Source: CAD feature listing. Evaluate the final solid. Frame: model axes, mm. A direction names the side the tool comes from. Coordinates: 2 decimals unless noted, no trailing zeros. Write each loop counter-clockwise with the first axis right and the second up, starting at its lowest first coordinate (ties: lowest second). Pieces come first, ordered by that corner, then holes. Notation, with made-up numbers: M -13,79.5 L 42,79.5 A5 ccw 42,87.5 Z; hole C 61,64 d6. An arc over 180 degrees is marked long. One line per item, written item: value. Start each with the question number.
Item 1: Set-up query: faces 3 (the flat face through (2.5, 7, 0)), 4 (the cylindrical face through (-1.494, 4.107, -10.965)), 5 (the cylindrical face through (55.608, -59.05, -11.462)). Return all of +Z, -Z, +X, -X, +Y, -Y with unobstructed straight access to the full face (end or side cutting, diameter ignored); none if empty.
Item 2: Ray query, L1, parallel to Y at x = 74.5, z = 15.5; L2, parallel to X at y = 37.5, z = -2; L3, parallel to Y at x = 18, z = -20. Return the intervals inside material, ascending. Write a range as from..to.
Item 3: Cut plane C-C, the plane x = 49. Output: boundary loops of the cut face in (y, z), then the cut area to 3 significant figures.
Item 4: Pin query (flat end, axial travel): P1, Ø3, axis at y = 7.5, z = 11.5, coming from the -X side; P2, Ø5, axis at x = 21.5, z = -2, coming from the +Y side; P3, Ø8, axis at x = 78.5, z = 17.5, coming from the +Y side. Return the tip coordinate at first contact, or that it passes through.
Item 5: Cut plane A-A, the plane y = -15.5. Output: boundary loops of the cut face in (x, z), then the cut area to 3 significant figures.
Item 6: Mould query, pull axis Z, two halves, no side actions, for faces 1 (the flat face through (60, -61.022, 0)), 2 (the flat face through (-1, 8, 9)). Classes: released by +Z, released by -Z, zero draft, split by the parting line, or undercut.
Item 7: Cut plane D-D, the plane z = -4. Output: boundary loops of the cut face in (x, y).
Item 8: Cut plane B-B, the plane z = 2. Output: boundary loops of the cut face in (x, y).
```python
from build123d import *

# Parameters (mm, degrees)
SKETCH_2_W                   = 5
SKETCH_2_H                   = 44
CUT_EXTRUDE_1_DEPTH          = 136.500823221
CUT_EXTRUDE_2_DEPTH          = 112.990773585
HOLE_WIZARD_M31_D            = 3
HOLE_WIZARD_M31_CSINK_D      = 5
HOLE_WIZARD_M31_CSINK_ANGLE  = 90
HOLE_WIZARD_M31_2_AT_2_COUNT = 2
HOLE_WIZARD_M31_2_AT_2_PITCH = 21.213203436
HOLE_WIZARD_M31_2_AT_3_COUNT = 2
HOLE_WIZARD_M31_2_AT_3_PITCH = 21.213203436
HOLE_WIZARD_M31_2_AT_4_COUNT = 2
HOLE_WIZARD_M31_2_AT_4_PITCH = 30


with BuildPart() as part:
    # По траектории1: sweep along a path in Эскиз1
    with BuildLine(Plane.XY) as sweep_1_path:
        Line((0, 43.940273354), (0, -28.521737175))
        ThreePointArc((0, -28.521737175), (8.786796564, -49.734940611), (30, -58.521737175))
        Line((30, -58.521737175), (66.792283136, -58.521737175))
        Line((66.792283136, -58.521737175), (88.792283136, -58.521737175))
    # Эскиз2 → По траектории1 (sweep)
    with BuildSketch(Plane(origin=(0, 0, 0), x_dir=(1, 0, 0), z_dir=(0, 1, 0))):
        Rectangle(SKETCH_2_W, SKETCH_2_H)
    sweep(path=sweep_1_path.line)

    # Эскиз3 → Вырез-Вытянуть1 (cut, through all)
    with BuildSketch(Plane(origin=(0, -56.021737175, 0), x_dir=(1, 0, 0), z_dir=(0, 1, 0))):
        with BuildLine():
            Line((88.792283136, 22), (66.792283136, 22))
            ThreePointArc((66.792283136, 22), (82.348632323, 15.556349186), (88.792283136, 0))
            Line((88.792283136, 0), (88.792283136, 22))
        make_face()
        with BuildLine():
            Line((88.792283136, -22), (88.792283136, 0))
            ThreePointArc((88.792283136, 0), (82.348632323, -15.556349186), (66.792283136, -22))
            Line((66.792283136, -22), (88.792283136, -22))
        make_face()
    extrude(amount=-CUT_EXTRUDE_1_DEPTH, mode=Mode.SUBTRACT)

    # Эскиз4 → Вырез-Вытянуть2 (cut, through all)
    with BuildSketch(Plane.ZY.offset(2.5)):
        with BuildLine():
            Line((22, 43.940273354), (-22, 43.940273354))
            Line((-22, 43.940273354), (-22, 31.296679815))
            ThreePointArc((-22, 31.296679815), (0, 43.440273354), (22, 31.296679815))
            Line((22, 31.296679815), (22, 43.940273354))
        make_face()
    extrude(amount=-CUT_EXTRUDE_2_DEPTH, mode=Mode.SUBTRACT)

    # Hole Wizard M31 (through all)
    with Locations(Plane(origin=(0, -56.021737175, 0), x_dir=(1, 0, 0), z_dir=(0, 1, 0))):
        with Locations((54.417914466, -12.374368671), (79.166651807, -12.374368671), (79.166651807, 12.374368671), (54.417914466, 12.374368671)):
            CounterSinkHole(HOLE_WIZARD_M31_D / 2, HOLE_WIZARD_M31_CSINK_D / 2, counter_sink_angle=HOLE_WIZARD_M31_CSINK_ANGLE)

    # Эскиз10 → Hole Wizard M31 2 (revolve, cut)
    with BuildSketch(Plane(origin=(-2.5, 28.046875072, -10.606601718), x_dir=(0, 0, 1), z_dir=(0, 1, 0))):
        Polygon((0, 0), (0, 91.292283136), (1.5, 91.292283136), (1.5, 1.5), (2.75, 1.5), (2.75, 0.525), (3.275, 0), align=None)
    hole_wizard_m31_2 = revolve(axis=Axis((-8.85, 28.046875072, -10.606601718), (1, 0, 0)), mode=Mode.SUBTRACT)

    # Hole Wizard M31 2 at 2: Hole Wizard M31 2 ×2
    with Locations(*[(0, 0, i * HOLE_WIZARD_M31_2_AT_2_PITCH) for i in range(1, HOLE_WIZARD_M31_2_AT_2_COUNT)]):
        add(hole_wizard_m31_2, mode=Mode.SUBTRACT)

    # Hole Wizard M31 2 at 3: Hole Wizard M31 2 ×2
    with Locations(*[(0, -i * HOLE_WIZARD_M31_2_AT_3_PITCH, 0) for i in range(1, HOLE_WIZARD_M31_2_AT_3_COUNT)]):
        add(hole_wizard_m31_2, mode=Mode.SUBTRACT)

    # Hole Wizard M31 2 at 4: Hole Wizard M31 2 ×2
    with Locations(*[Vector(0, -0.7071067811865492, 0.7071067811865459) * (i * HOLE_WIZARD_M31_2_AT_4_PITCH) for i in range(1, HOLE_WIZARD_M31_2_AT_4_COUNT)]):
        add(hole_wizard_m31_2, mode=Mode.SUBTRACT)


solid = part.part
```
From the geometry:
1. face 3: +Z, -Z, +X, +Y
1. face 4: -X
1. face 5: +Y, -Y
2. L1: y = -61.02..-56.02
2. L2: x = -2.5..2.5
2. L3: y = -58.73..-53.27
3. outline: M -61.02,-22 L -56.02,-22 L -56.02,22 L -61.02,22 Z
3. area: 220 mm²
4. P1: stops at x = -1
4. P2: stops at y = -53.73
4. P3: stops at y = -56.02
5. outline: M -2.5,-22 L 2.5,-22 L 2.5,22 L -2.5,22 Z
5. area: 220 mm²
6. face 1: zero draft
6. face 2: undercut
7. outline: M -2.5,-28.52 A32.5 ccw 30,-61.02 L 88.43,-61.02 L 88.43,-56.02 L 30,-56.02 A27.5 cw 2.5,-28.52 L 2.5,43.13 L -2.5,43.13 Z
8. outline: M -2.5,-28.52 A32.5 ccw 30,-61.02 L 88.7,-61.02 L 88.7,-56.02 L 30,-56.02 A27.5 cw 2.5,-28.52 L 2.5,43.36 L -2.5,43.36 Z
